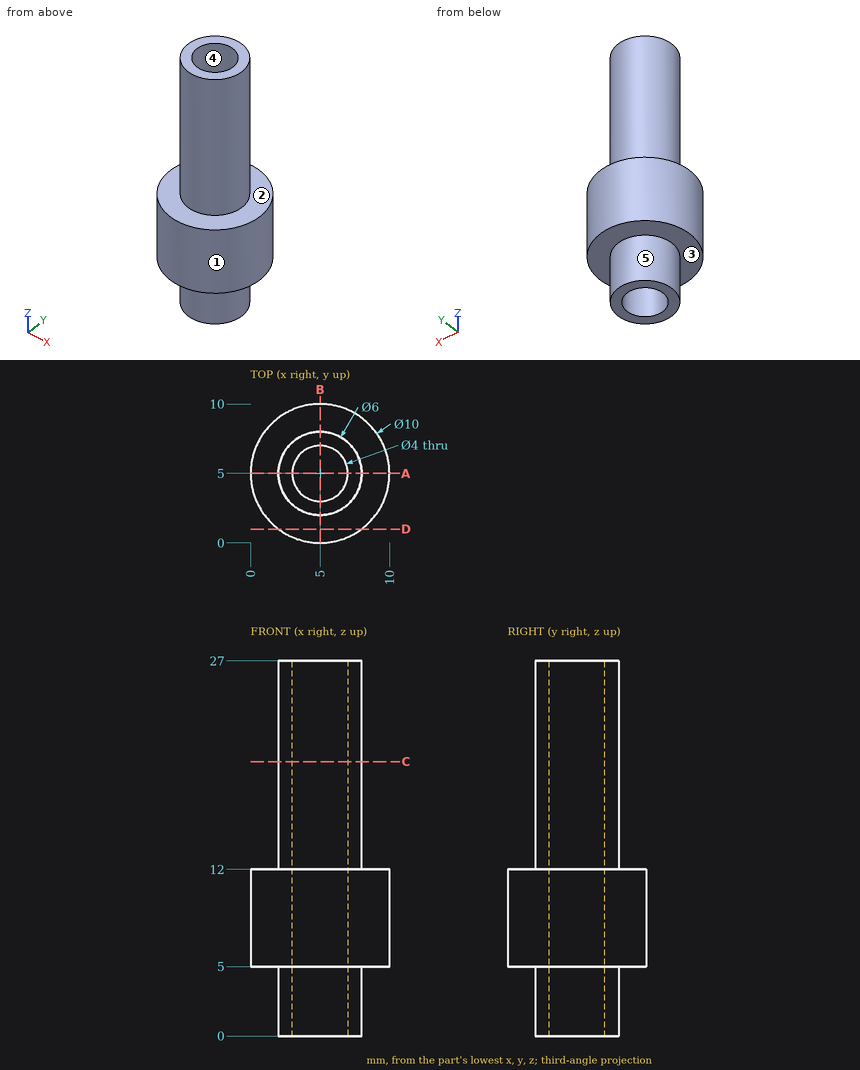
Can you work these out from the drawing? Everything is in mm from the part's minimum corner. A direction names the side the tool comes from. Round coordinates to 2 decimals unless told otherwise and drop trailing zeros. Write each loop counter-clockwise with the first axis right and the second up, starting at its lowest first coordinate (ties: lowest second). Pieces come first, ordered by that corner, then holes.
1. Will these pins go through, and if not, where does the flat tip stop? pin 1 Ø1 at (x, y) = (1, 7) entering from +Z; pin 2 Ø1.5 at (x, z) = (8, 3) entering from +Y; pin 3 Ø3 at (y, z) = (3, 12.5) entering from -X.
2. Suppose I cut it at A-A (y = 5). List the corners of the cut face in (x, z) for me.
3. Suppose I cut it at D-D (y = 1). List the corners of the cut face in (x, z) for me.
4. If we mould it in two halves opening along Y, with no side actions, what happens to the marked faces 3, 4 and 5? For each: released by +Y, released by -Y, zero draft, split by the parting line, or undercut.
5. For the marked faces 1 and 2, which set-ups out of +Z, -Z, +X, -X, +Y, -Y let a thin tool reach every point of the face, with its end or its side?
6. Suppose I cut it at C-C (z = 19.75). List the corners of the cut face in (x, y) for me, and give its area (3 significant figures).
7. I need wall thicknesses on L1, parallel to Y at x = 5, z = 20; L2, parallel to Z at x = 2.5, y = 1; L3, parallel to Y at x = 5, z = 8.75. Which ranges of each line are inside material? Lowest first, please.
Answer sheet:
1. pin 1: stops at z = 12
1. pin 2: stops at y = 6.98
1. pin 3: stops at x = 0.03
2. outline: (0, 5) - (2, 5) - (2, 0) - (3, 0) - (3, 27) - (2, 27) - (2, 12) - (0, 12) - close; (7, 0) - (8, 0) - (8, 5) - (10, 5) - (10, 12) - (8, 12) - (8, 27) - (7, 27) - close
3. outline: (2, 5) - (8, 5) - (8, 12) - (2, 12) - close
4. face 3: zero draft
4. face 4: undercut
4. face 5: split by the parting line
5. face 1: +Z, -Z
5. face 2: +Z
6. outline: circle Ø6 at (5, 5); hole circle Ø4 at (5, 5)
6. area: 15.7 mm2
7. L1: y = 2 to 3, 7 to 8
7. L2: z = 5 to 12
7. L3: y = 0 to 3, 7 to 10
